```python
from build123d import *

# Parameters (mm, degrees)
SKETCH1_R           = 7.8105
BOSS_EXTRUDE1_DEPTH = 10.16
CHAMFER2_SIZE       = 0.635
SKETCH2_R           = 1.5875
CUT_EXTRUDE1_DEPTH  = 34.335322786


with BuildPart() as part:
    # Sketch1 → Boss-Extrude1 (new body)
    with BuildSketch(Plane.XY):
        with BuildLine():
            Line((4.5, 4.699), (-4.5, 4.699))
            Line((-4.5, 4.699), (-4.5, 0))
            Line((-4.5, 0), (-15.875, 0))
            Line((-15.875, 0), (-15.875, 11.6205))
            Line((-15.875, 11.6205), (-11.6205, 15.875))
            ThreePointArc((-11.6205, 15.875), (0, 27.4955), (11.6205, 15.875))
            Line((11.6205, 15.875), (15.875, 11.6205))
            Line((15.875, 11.6205), (15.875, 0))
            Line((15.875, 0), (4.5, 0))
            Line((4.5, 0), (4.5, 4.699))
        make_face()
        with Locations((0, 15.875)):
            Circle(SKETCH1_R, mode=Mode.SUBTRACT)
    extrude(amount=BOSS_EXTRUDE1_DEPTH)

    # Chamfer2
    chamfer2_edges = [part.edges().sort_by_distance(p)[0] for p in [
        (-13.74775, 13.74775, 0),
        (0, 27.4955, 0),
        (13.74775, 13.74775, 0),
        (15.875, 5.81025, 0),
        (15.875, 5.81025, 10.16),
        (13.74775, 13.74775, 10.16),
        (0, 27.4955, 10.16),
        (-13.74775, 13.74775, 10.16),
        (-15.875, 5.81025, 10.16),
        (-15.875, 5.81025, 0),
    ]]
    chamfer(chamfer2_edges, length=CHAMFER2_SIZE)

    # Sketch2 → Cut-Extrude1 (cut, through all)
    with BuildSketch(Plane.XY.offset(10.16)):
        with Locations((-12.7, 3.175)):
            Circle(SKETCH2_R)
        with Locations(Location((12.7, 3.175, 0), (0, 0, 180))):
            Circle(SKETCH2_R)
    extrude(amount=-CUT_EXTRUDE1_DEPTH, mode=Mode.SUBTRACT)


solid = part.part
```
Source: CAD feature listing. Evaluate the final solid. Frame: model axes, mm. A direction names the side the tool comes from. Round coordinates to 2 decimals unless told otherwise and drop trailing zeros. Loops run counter-clockwise (first coordinate to the right, second up) from the corner with the lowest first, then second, coordinate; pieces in that order, holes last.
1. Ray query, L1, parallel to Y at x = 0, z = 2.5; L2, parallel to Y at x = -7, z = 2.25; L3, parallel to X at y = 3, z = 3.5 (3 decimals). Return the intervals inside material, ascending.
2. Contact query for a flat-ended pin moving along its axis: pin 1 (1.5 mm diameter, centred on x = 1, z = 1.5, fed in from +Y). Output: stop coordinate, or through.
3. Access query for faces 1 (the cylindrical face through (-1.69, 8.25, 5.01)), 2 (the flat face through (-4.5, 2, 5)). Directions: +Z, -Z, +X, -X, +Y, -Y. A direction counts if a zero-diameter tool reaches every point of the face in a straight line with its end or side. Return the directions, or none.
4. Section query D-D on x = 12.7. Output: boundary loops of the cut face in (y, z) (1 decimal), and give its area (3 significant figures).
5. Mould query, pull axis Y, two halves, no side actions, for faces 3 (the flat face through (15.875, 6, 5)), 4 (the flat face through (13.394, 13.646, 9.847)), 5 (the cylindrical face through (-11.2, 3.7, 5.2)), 6 (the flat face through (-10, 0, 5)). Classes: released by +Y, released by -Y, zero draft, split by the parting line, or undercut.
6. Section query A-A on y = 8.5. Output: boundary loops of the cut face in (x, z) (3 decimals).
7. Section query B-B on x = 0. Output: boundary loops of the cut face in (y, z) (1 decimal).
8. Section query C-C on z = 8.25. Output: boundary loops of the cut face in (x, y) (1 decimal), and give its area (3 significant figures).
Answers below:
1. L1: y = 4.7 to 8.06, 23.69 to 27.5
1. L2: y = 0 to 12.41, 19.34 to 25.15
1. L3: x = -15.875 to -14.278, -11.122 to -4.5, 4.5 to 11.122, 14.278 to 15.875
2. pin 1: stops at y = 27.49
3. face 1: +Z, -Z
3. face 2: +Z, -Z, -Y
4. outline: (0, 0) - (1.6, 0) - (1.6, 10.2) - (0, 10.2) - close; (4.8, 0) - (13.9, 0) - (14.8, 0.6) - (14.8, 9.5) - (13.9, 10.2) - (4.8, 10.2) - close
4. area: 117 mm2
5. face 3: zero draft
5. face 4: released by +Y
5. face 5: undercut
5. face 6: released by -Y
6. outline: (-15.875, 0.635) - (-15.24, 0) - (-2.572, 0) - (-2.572, 10.16) - (-15.24, 10.16) - (-15.875, 9.525) - close; (2.572, 0) - (15.24, 0) - (15.875, 0.635) - (15.875, 9.525) - (15.24, 10.16) - (2.572, 10.16) - close
7. outline: (4.7, 0) - (8.1, 0) - (8.1, 10.2) - (4.7, 10.2) - close; (23.7, 0) - (26.9, 0) - (27.5, 0.6) - (27.5, 9.5) - (26.9, 10.2) - (23.7, 10.2) - close
8. outline: (-15.9, 0) - (-4.5, 0) - (-4.5, 4.7) - (4.5, 4.7) - (4.5, 0) - (15.9, 0) - (15.9, 11.6) - (11.6, 15.9) arc R11.6 ccw to (-11.6, 15.9) - (-15.9, 11.6) - close; hole circle Ø3.2 at (-12.7, 3.2); hole circle Ø15.6 at (0, 15.9); hole circle Ø3.2 at (12.7, 3.2)
8. area: 448 mm2
